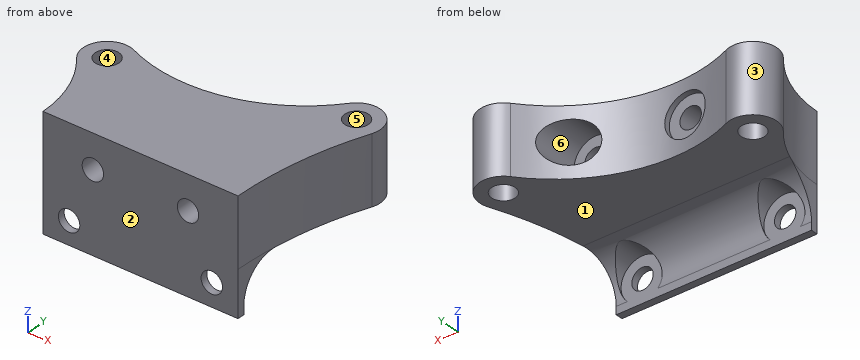
from build123d import *

# Parameters (mm, degrees)
SZKIC1_R                                            = 5
DODANIE_WYCI_GNI_CIE1_DEPTH                         = 28.7
DODANIE_WYCI_GNI_CIE2_REACH                         = 120.092
DODANIE_WYCI_GNI_CIE2_END_RADIUS                    = 50.543324632
WYTNIJ_WYCI_GNI_CIE1_START                          = -19.3
WYTNIJ_WYCI_GNI_CIE1_DEPTH                          = 19.3
POG_BIENIE_WALCOWE_POD_M8_WKR_T_Z_BEM_S_D           = 9
POG_BIENIE_WALCOWE_POD_M8_WKR_T_Z_BEM_S_CBORE_D     = 18.011
POG_BIENIE_WALCOWE_POD_M8_WKR_T_Z_BEM_S_CBORE_DEPTH = 20.3
POG_BIENIE_WALCOWE_POD_M8_WKR_T_Z_B_2_D             = 9
POG_BIENIE_WALCOWE_POD_M8_WKR_T_Z_B_2_CBORE_D       = 18.011
POG_BIENIE_WALCOWE_POD_M8_WKR_T_Z_B_2_CBORE_DEPTH   = 57.54


with BuildPart() as part:
    # Szkic1 → Dodanie-wyciągnięcie1 (new body)
    with BuildSketch(Plane.XY):
        with BuildLine():
            Line((-1.469986393, -60.54), (-83.469986393, -60.54))
            ThreePointArc((-83.469986393, -60.54), (-86.43214098, -43.49124867), (-94.971403209, -28.440824015))
            ThreePointArc((-94.971403209, -28.440824015), (-95.242829308, -16.084497343), (-83.300365534, -12.901724973))
            ThreePointArc((-83.300365534, -12.901724973), (-42.333721248, -16.139046942), (-7.843535904, 6.203139892))
            ThreePointArc((-7.843535904, 6.203139892), (4.984530504, 8.669166953), (9.306965288, -3.657922516))
            ThreePointArc((9.306965288, -3.657922516), (1.248004894, -31.593007814), (-1.469986393, -60.54))
        make_face()
        with Locations((-87.246959259, -22.09)):
            Circle(SZKIC1_R, mode=Mode.SUBTRACT)
        Circle(SZKIC1_R, mode=Mode.SUBTRACT)
    extrude(amount=DODANIE_WYCI_GNI_CIE1_DEPTH)

    # Dodanie-wyciągnięcie2: up to this cylinder (the profile starts outside it)
    dodanie_wyci_gni_cie2_end = Plane(origin=(-134.013311026, -60.54, -6.691691), z_dir=(0, 0, -1)) * Cylinder(DODANIE_WYCI_GNI_CIE2_END_RADIUS, 342.270649265, mode=Mode.PRIVATE)
    # Szkic3 → Dodanie-wyciągnięcie2 (add, up to the surface)
    with BuildSketch(Plane(origin=(0, 0, 0), x_dir=(0, 0, -1), z_dir=(1, 0, 0)), mode=Mode.PRIVATE) as dodanie_wyci_gni_cie2_sk1:
        with BuildLine():
            Line((0, -60.54), (0, -41.54))
            ThreePointArc((0, -41.54), (4.686291501, -52.853708499), (16, -57.54))
            Line((16, -57.54), (19.3, -57.54))
            Line((19.3, -57.54), (19.3, -60.54))
            Line((19.3, -60.54), (0, -60.54))
        make_face()
    dodanie_wyci_gni_cie2_tool1 = extrude(dodanie_wyci_gni_cie2_sk1.sketch, amount=-DODANIE_WYCI_GNI_CIE2_REACH, mode=Mode.PRIVATE) - dodanie_wyci_gni_cie2_end
    add(dodanie_wyci_gni_cie2_tool1.solids().sort_by_distance((0, -56.56965, -6.691691))[0])

    # Szkic4 → Wytnij-wyciągnięcie1 (cut)
    with BuildSketch(Plane.XY.offset(WYTNIJ_WYCI_GNI_CIE1_START)):
        with BuildLine():
            Line((-1.469986393, -60.54), (0, -60.54))
            Line((0, -60.54), (0, -41.54))
            Line((0, -41.54), (-0.304878126, -41.54))
            ThreePointArc((-0.304878126, -41.54), (-1.178436016, -51.022155217), (-1.469986393, -60.54))
        make_face()
    extrude(amount=WYTNIJ_WYCI_GNI_CIE1_DEPTH, mode=Mode.SUBTRACT)

    # Pog_bienie walcowe pod M8 Wkr_t z _bem s (through all)
    with Locations(Plane(origin=(0, 0, 0), x_dir=(1, 0, 0), z_dir=(0, 1, 0))):
        with Locations((-62.500071487, -14.35), (-22.500071487, -14.35)):
            CounterBoreHole(POG_BIENIE_WALCOWE_POD_M8_WKR_T_Z_BEM_S_D / 2, POG_BIENIE_WALCOWE_POD_M8_WKR_T_Z_BEM_S_CBORE_D / 2, POG_BIENIE_WALCOWE_POD_M8_WKR_T_Z_BEM_S_CBORE_DEPTH)

    # Pog_bienie walcowe pod M8 Wkr_t z _b 2 (through all)
    with Locations(Plane(origin=(0, 0, 0), x_dir=(1, 0, 0), z_dir=(0, 1, 0))):
        with Locations((-72.500071487, 9.65), (-12.500071487, 9.65)):
            CounterBoreHole(POG_BIENIE_WALCOWE_POD_M8_WKR_T_Z_B_2_D / 2, POG_BIENIE_WALCOWE_POD_M8_WKR_T_Z_B_2_CBORE_D / 2, POG_BIENIE_WALCOWE_POD_M8_WKR_T_Z_B_2_CBORE_DEPTH)


solid = part.part
Could you check a few things on this model? Use its own coordinates, in mm. Face numbers are marked on the shaded views. A direction names the side the tool comes from. Round coordinates to 2 decimals unless told otherwise and drop trailing zeros. Write each loop counter-clockwise with the first axis right and the second up, starting at its lowest first coordinate (ties: lowest second). Pieces come first, ordered by that corner, then holes. Notation, with made-up numbers: (76.25, 13) - (89.25, 13) arc R23 ccw to (89.25, 23) - close; hole circle Ø1 at (83, 38). An arc over 180 degrees is marked (long way). Use a Markdown table: item, result.
Q1. I want a section at A-A (z = 14.35). List the corners of the cut face in (x, y) for me (3 decimals).
Output values:
| item | result |
|---|---|
| outline | (-94.971, -28.441) arc R50.543 cw to (-83.47, -60.54) - (-67, -60.54) - (-67, -20.3) - (-71.506, -20.3) - (-71.506, -16.665) arc R64 cw to (-83.3, -12.902) arc R10 ccw to start; (-58, -60.54) - (-27, -60.54) - (-27, -20.3) - (-31.506, -20.3) - (-31.506, -12.336) arc R64 cw to (-53.495, -17.935) - (-53.495, -20.3) - (-58, -20.3) - close; (-18, -60.54) - (-1.47, -60.54) arc R155.504 cw to (9.307, -3.658) arc R10 ccw to (-7.844, 6.203) arc R64 cw to (-13.495, -0.048) - (-13.495, -20.3) - (-18, -20.3) - close; hole circle Ø10 at (-87.247, -22.09); hole circle Ø10 at (0, 0) |
Q2. Thinking about a two-plate mould opening in Y: for the marked faces 1, 2, 3 and 4, which applies, released by +Y, released by -Y, zero draft, split by the parting line, or undercut?
Output values:
| item | result |
|---|---|
| face 1 | zero draft |
| face 2 | released by -Y |
| face 3 | split by the parting line |
| face 4 | undercut |
Q3. I want a section at D-D (z = -11.5). List the corners of the cut face in (x, y) for me, plus the area to 3 significant figures.
Output values:
| item | result |
|---|---|
| outline | (-83.6, -56.89) arc R50.54 cw to (-83.47, -60.54) - (-76.6, -60.54) - (-76.6, -57.54) - (-81.31, -57.54) - (-81.31, -56.89) - close; (-68.4, -60.54) - (-16.6, -60.54) - (-16.6, -57.54) - (-21.31, -57.54) - (-21.31, -56.89) - (-63.69, -56.89) - (-63.69, -57.54) - (-68.4, -57.54) - close; (-8.4, -60.54) - (-1.47, -60.54) arc R155.5 cw to (-1.43, -56.89) - (-3.69, -56.89) - (-3.69, -57.54) - (-8.4, -57.54) - close |
| area | 227 mm2 |
Q4. For pin 1 (13 mm diameter, centred on x = -87.25, y = -22.09, fed in from -Z); pin 2 (6 mm diameter, centred on x = 0, y = 0, fed in from +Z); pin 3 (16 mm diameter, centred on x = -62.5, z = 14.35, fed in from +Y); pin 4 (12 mm diameter, centred on x = -82, z = -5, fed in from +Y), each with a flat end and sliding along its axis, tell me the tip position at first contact or that it passes through.
Output values:
| item | result |
|---|---|
| pin 1 | z = 0 |
| pin 2 | through |
| pin 3 | y = -20.3 |
| pin 4 | y = -12.28 |
Q5. I want a section at C-C (x = -23). List the corners of the cut face in (y, z) for me, plus the area to 3 significant figures.
Output values:
| item | result |
|---|---|
| outline | (-60.54, -19.3) - (-57.54, -19.3) - (-57.54, -16) arc R16 cw to (-41.54, 0) - (-7.65, 0) - (-7.65, 5.36) - (-20.3, 5.36) - (-20.3, 9.88) - (-60.54, 9.88) - close; (-60.54, 18.82) - (-20.3, 18.82) - (-20.3, 23.34) - (-7.65, 23.34) - (-7.65, 28.7) - (-60.54, 28.7) - close |
| area | 1,040 mm2 |
Q6. I want a section at B-B (y = -22.09). List the corners of the cut face in (x, z) for me.
Output values:
| item | result |
|---|---|
| outline | (-97.25, 0) - (-92.25, 0) - (-92.25, 28.7) - (-97.25, 28.7) - close; (-82.25, 0) - (3.36, 0) - (3.36, 28.7) - (-82.25, 28.7) - close; hole circle Ø9 at (-62.5, 14.35); hole circle Ø9 at (-22.5, 14.35) |
Q7. For the marked faces 5 and 6, which set-ups out of +Z, -Z, +X, -X, +Y, -Y let a thin tool reach every point of the face, with its end or its side?
Output values:
| item | result |
|---|---|
| face 5 | +Z, -Z |
| face 6 | +Y |
Q8. Please list where these lines run through material, in increasing order: L1, parallel to Z at x = -83.5, y = -51.5; L2, parallel to Y at x = -17, z = 9.5; L3, parallel to X at y = -20.5, z = 27.5.
Output values:
| item | result |
|---|---|
| L1 | -3.48 to 28.7 |
| L2 | -60.54 to -20.3 |
| L3 | -97.12 to -91.99, -82.51 to 3.77 |
